Check sheet for the drawn part. Datum: minimum x, y, z corner. Units: mm. Round coordinates to 2 decimals unless told otherwise and drop trailing zeros. Order: outer loops, then holes, each group sorted by start corner. A loop starts at its lowest first (then second) coordinate and runs counter-clockwise, first axis right, second up. Notation, with made-up numbers: (-8.75, 30.5) - (15.25, 30.5) arc R13 ccw to (15.25, 41.5) - close; hole circle Ø3 at (70.25, 62). An arc over 180 degrees is marked (long way). Write each question's results on one line, items separated by ' | '.
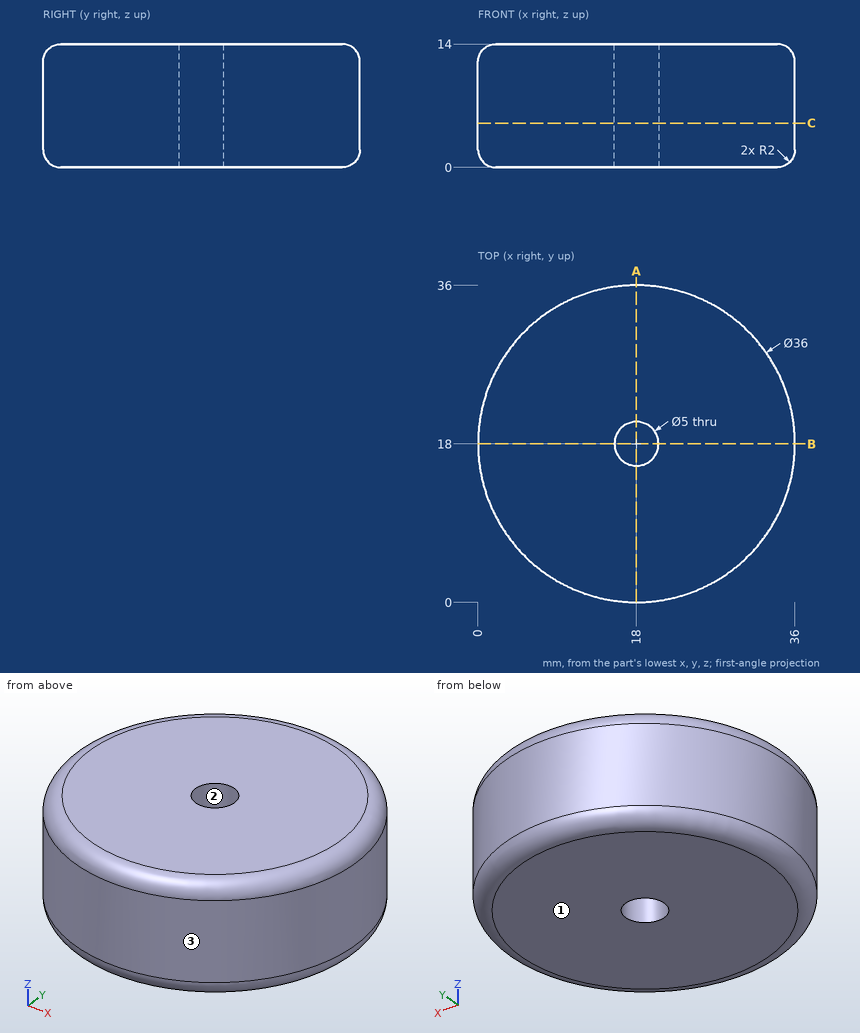
(1) Section check A-A (x = 18). Record the cut outline in (y, z).
Answers follow:
outline: (0, 2) arc R2 ccw to (2, 0) - (15.5, 0) - (15.5, 14) - (2, 14) arc R2 ccw to (0, 12) - close; (20.5, 0) - (34, 0) arc R2 ccw to (36, 2) - (36, 12) arc R2 ccw to (34, 14) - (20.5, 14) - close
(2) Section check C-C (z = 5). Record the cut outline in (x, y).
Answers follow:
outline: circle Ø36 at (18, 18); hole circle Ø5 at (18, 18)
(3) Material ranges on line 1 (Y direction, x = 18, z = 6); line 2 (Y direction, x = 16, z = 7.75); line 3 (X direction, y = 4, z = 5.25), recorded low to high.
Answers follow:
line 1: 0 to 15.5, 20.5 to 36 | line 2: 0.11 to 16.5, 19.5 to 35.89 | line 3: 6.69 to 29.31
(4) Depth check by flat-ended pin: pin 1 Ø4 at (y, z) = (31.5, 5.5) entering from -X; pin 2 Ø4 at (x, z) = (18, 11) entering from -Y; pin 3 Ø1 at (x, z) = (31.5, 6) entering from +Y. Enter the tip coordinate at first touch or a pass-through.
Answers follow:
pin 1: x = 4.15 | pin 2: y = 0 | pin 3: y = 30.45
(5) Draft check along Y on the marked faces 1, 2 and 3. Enter one of: released by +Y, released by -Y, zero draft, split by the parting line, or undercut.
Answers follow:
face 1: zero draft | face 2: undercut | face 3: split by the parting line
